Check sheet for the modelled part. Datum: model origin and axes. Units: mm. Face numbers are marked on the shaded views. Give positions to 0.01 mm unless a question says otherwise; leave off trailing zeros. Order: outer loops, then holes, each group sorted by start corner. A loop starts at its lowest first (then second) coordinate and runs counter-clockwise, first axis right, second up.
Item 1: Sectioned sample at D-D on x = -24. Record the boundary of the cut face in (y, z).
Item 2: Sectioned sample at C-C on z = 114.3. Record the boundary of the cut face in (x, y), and give its area (3 significant figures).
Item 3: Sectioned sample at B-B on x = -114.3. Record the boundary of the cut face in (y, z).
Item 4: Release check for a two-part mould opening along X. For the marked faces 1, 2, 3 and 4 record: released by +X, released by -X, zero draft, split by the parting line, or undercut.
Item 5: Sectioned sample at A-A on z = 0. Record the boundary of the cut face in (x, y) (1 decimal), and give its area (3 significant figures).
Item 6: Material ranges on line 1 along Z through (x, y) = (0, 0.5) (1 decimal); line 2 along Z through (x, y) = (4.5, 5.5); line 3 along Z through (x, y) = (-26, 19.5) (3 decimals), recorded low to high.
Item 7: Gauge pin test, flat ends, axial feed: P1, Ø8, axis at x = 59.5, y = 5.5, coming from the -Z side; P2, Ø1, axis at y = 18.5, z = -102, coming from the -X side; P3, Ø12.5, axis at x = 0, z = 0, coming from the +Y side. Record the tip position at first contact, or that the pin passes through.
from build123d import *

# Parameters (mm, degrees)
F2_R     = 4.7625
F3_DEPTH = 1.017


with BuildPart() as f1:
    # F0 (on Top) → F1 (revolve)
    with BuildSketch(Plane.XY):
        Polygon((0, 1.016), (0, 0), (130.175, 0), (130.175, 25.4), (129.159, 25.4), (129.159, 1.016), align=None)
    revolve(axis=Axis((0, 0.508, 0), (0, 1, 0)))

    # F2 (on face) → F3 (cut, through all)
    with BuildSketch(Plane(origin=(0, 1.016, 0), x_dir=(-1, 0, 0), z_dir=(0, 1, 0))):
        Circle(F2_R)
        with Locations((0, -50.8)):
            Circle(F2_R)
        with Locations((0, -114.3)):
            Circle(F2_R)
        with Locations((-50.8, 0)):
            Circle(F2_R)
        with Locations((0, 50.8)):
            Circle(F2_R)
        with Locations((-80.822305, 80.822305)):
            Circle(F2_R)
        with Locations((80.822305, 80.822305)):
            Circle(F2_R)
        with Locations((114.3, 0)):
            Circle(F2_R)
        with Locations((80.822305, -80.822305)):
            Circle(F2_R)
        with Locations((-80.822305, -80.822305)):
            Circle(F2_R)
        with Locations((0, 114.3)):
            Circle(F2_R)
        with Locations((50.8, 0)):
            Circle(F2_R)
        with Locations((-114.3, 0)):
            Circle(F2_R)
    extrude(amount=-F3_DEPTH, mode=Mode.SUBTRACT)


solid = f1.part
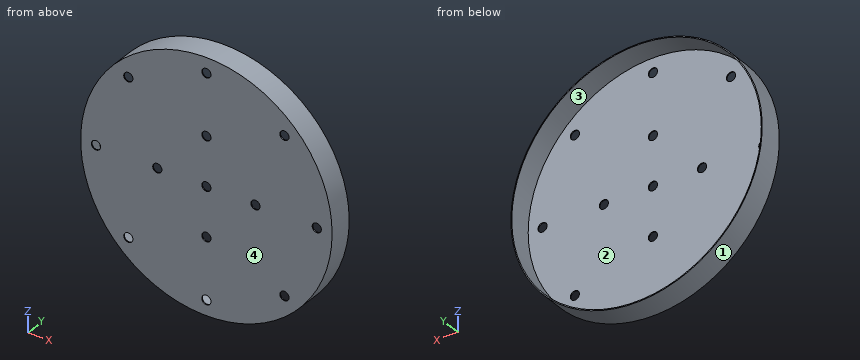
Report:
1. outline: (0, -127.94) - (25.4, -127.94) - (25.4, -126.91) - (1.02, -126.91) - (1.02, 126.91) - (25.4, 126.91) - (25.4, 127.94) - (0, 127.94) - close
2. outline: (-62.3, 0) - (-4.76, 0) - (-4.76, 1.02) - (-60.15, 1.02) - (-60.15, 25.4) - (-62.3, 25.4) - close; (4.76, 0) - (62.3, 0) - (62.3, 25.4) - (60.15, 25.4) - (60.15, 1.02) - (4.76, 1.02) - close
2. area: 222 mm2
3. outline: (0, -62.3) - (25.4, -62.3) - (25.4, -60.15) - (1.02, -60.15) - (1.02, -4.76) - (0, -4.76) - close; (0, 4.76) - (1.02, 4.76) - (1.02, 60.15) - (25.4, 60.15) - (25.4, 62.3) - (0, 62.3) - close
4. face 1: split by the parting line
4. face 2: undercut
4. face 3: undercut
4. face 4: zero draft
5. outline: (-130.2, 0) - (-119.1, 0) - (-119.1, 1) - (-129.2, 1) - (-129.2, 25.4) - (-130.2, 25.4) - close; (-109.5, 0) - (-55.6, 0) - (-55.6, 1) - (-109.5, 1) - close; (-46, 0) - (-4.8, 0) - (-4.8, 1) - (-46, 1) - close; (4.8, 0) - (46, 0) - (46, 1) - (4.8, 1) - close; (55.6, 0) - (109.5, 0) - (109.5, 1) - (55.6, 1) - close; (119.1, 0) - (130.2, 0) - (130.2, 25.4) - (129.2, 25.4) - (129.2, 1) - (119.1, 1) - close
5. area: 266 mm2
6. line 1: z = -130.2 to -119.1, -109.5 to -55.6, -46 to -4.8, 4.8 to 46, 55.6 to 109.5, 119.1 to 130.2
6. line 2: z = -130.1 to -129.08, 129.08 to 130.1
6. line 3: z = -127.552 to -126.515, 126.515 to 127.552
7. P1: stops at z = -117.75
7. P2: stops at x = -81.51
7. P3: stops at y = 1.02
